```python
from build123d import *

# Parameters (mm, degrees)
SKETCH_1_W     = 8
SKETCH_1_H     = 1.75
CHAMFER_1_SIZE = 0.1


with BuildPart() as part:
    # 草图1 → 旋转1 (revolve)
    with BuildSketch(Plane.XY):
        with Locations((0, 0.875)):
            Rectangle(SKETCH_1_W, SKETCH_1_H)
    revolve(axis=Axis((-4, 0, 0), (1, 0, 0)))

    # 草图3 → Hole Wizard 380 (revolve, cut)
    with BuildSketch(Plane(origin=(-4, 0, 0), x_dir=(0, 0, 1), z_dir=(0, 1, 0))):
        Polygon((0, 0), (0, 6.480688495), (0.8, 6), (0.8, 0), align=None)
    hole_wizard_380 = revolve(axis=Axis((-10.35, 0, 0), (1, 0, 0)), mode=Mode.SUBTRACT)

    # 镜向1: Hole Wizard 380 across plane
    add(hole_wizard_380.mirror(Plane(origin=(0, 0, 0), x_dir=(0, 0, 1), z_dir=(1, 0, 0))), mode=Mode.SUBTRACT)

    # 倒角1
    chamfer_1_edges = [part.edges().sort_by_distance(p)[0] for p in [
        (-4, -1.75, 0),
        (4, -1.75, 0),
    ]]
    chamfer(chamfer_1_edges, length=CHAMFER_1_SIZE)


solid = part.part
```
For this review, take the finished solid that the model builds, in its own axes (mm). Coordinates: 2 decimals unless noted, no trailing zeros. Loops run counter-clockwise (first coordinate to the right, second up) from the corner with the lowest first, then second, coordinate; pieces in that order, holes last. Notation, with made-up numbers: (29, 68.25) -> (70, 68.25) arc R16 ccw to (70, 74.25) -> close; hole circle Ø11 at (-21, -29). An arc over 180 degrees is marked (long way). Return JSON: item names as keys, results as strings. Group by question number.
(1) For pin 1 Ø1 at (x, z) = (-1, -1) entering from -Y; pin 2 Ø1 at (y, z) = (0, 0) entering from -X, all flat-tipped, find the tip position at first contact; note any pin that passes through.
(2) Consider section C-C, the plane x = -1.25. Give the boundary of the cut face in (y, z).
(3) To check wall thickness, follow L1, parallel to Z at x = -3.2, y = 0; L2, parallel to Z at x = -1, y = 0.5; L3, parallel to Y at x = 3.75, z = -0.1. State the ranges of each line that lie inside material, in increasing order.
(4) Consider section A-A, the plane z = 0. Give the boundary of the cut face in (x, y), plus the area to 3 significant figures.
Results below:
{
 "1": {"pin 1": "stops at y = -1.68", "pin 2": "passes through"},
 "2": {"outline": "circle Ø3.5 at (0, 0); hole circle Ø1.6 at (0, 0)"},
 "3": {"L1": "z = -1.75 to -0.8, 0.8 to 1.75", "L2": "z = -1.68 to -0.62, 0.62 to 1.68", "L3": "y = -1.75 to -0.79, 0.79 to 1.75"},
 "4": {"outline": "(-4, -1.65) -> (-3.9, -1.75) -> (3.9, -1.75) -> (4, -1.65) -> (4, -0.8) -> (-4, -0.8) -> close; (-4, 0.8) -> (4, 0.8) -> (4, 1.65) -> (3.9, 1.75) -> (-3.9, 1.75) -> (-4, 1.65) -> close", "area": "15.2 mm2"}
}
